Autodesk Inventor part; units mm, degrees
ref_plane "YZ Plane" through (0, 0, 0) normal (1, 0, 0) x (0, 1, 0)
ref_plane "XZ Plane" through (0, 0, 0) normal (0, 1, 0) x (-1, 0, 0)
ref_plane "XY Plane" through (0, 0, 0) normal (0, 0, 1) x (1, 0, 0)
sketch "Sketch1" plane through (0, 0, 0) normal (0, 1, 0) x (-1, 0, 0)
  circle A0 centre (0, 0) radius 66.5
  circle A1 centre (0, 0) radius 15
  dimension "d0" = 133
  dimension "d3" = 30
extrude "Extrusion2" add sketch "Sketch1" along normal blind 3
sketch "Sketch3" plane through (0, 3, 0) normal (0, 1, 0) x (1, 0, 0)
  circle A0 centre (0, 0) radius 66.5
  circle A1 centre (0, 0) radius 68.5
  dimension "d6" = 133
  dimension "d7" = 137
extrude "Extrusion3" add sketch "Sketch3" against normal blind 17
sketch "Sketch4" plane through (0, 0, 0) normal (0, -1, 0) x (1, 0, 0)
  circle A0 centre (0, 0) radius 15
  circle A1 centre (0, 0) radius 39
  line L0 (10.6103, -10.6029) -> (27.5808, -27.5735)
  line L1 (39, 0) -> (15, 0)
  circle A2 centre (0, 0) radius 15
  line L2 (27.7885, -27.3642) -> (10.8166, -10.3923)
  dimension "d10" = 30
  dimension "d11" = 24
extrude "Extrusion4" cut sketch "Sketch4" against normal blind 1.5 contours L1 A1 L2 A0 | A0 L2 A1 L0
mirror "Mirror1" about plane through (0, 0, 0) normal (0, 0, 1) of "Extrusion4"
fillet "Fillet1" radius 6 1 edges at (-68.5, 3, 0)
fillet "Fillet2" radius 2 1 edges at (-66.5, 0, 0)
properties part number "DireccionBase"
Geometry: final body of the model. Coordinates: model frame, mm. A direction names the side the tool comes from. Give positions to 0.01 mm unless a question says otherwise; leave off trailing zeros. Loops run counter-clockwise (first coordinate to the right, second up) from the corner with the lowest first, then second, coordinate; pieces in that order, holes last. Notation, with made-up numbers: (38, -13.75) -> (55, -13.75) arc R28 cw to (55, 4.25) -> close; hole circle Ø9 at (68.5, 78.25). An arc over 180 degrees is marked (long way). Put each result on its own line as item: value.
1. Set-up query: faces 4 (the cylindrical face through (-13.856, 1.479, 5.745)), 5 (the flat face through (25, 1.5, 0)). Return all of +Z, -Z, +X, -X, +Y, -Y with unobstructed straight access to the full face (end or side cutting, diameter ignored); none if empty.
Taken from the geometry:
face 4: +Y, -Y
face 5: -Y
2. Pin query (flat end, axial travel): P1, Ø8, axis at x = -37, y = -2.5, coming from the +Z side; P2, Ø5, axis at x = -39.5, y = -4.5, coming from the +Z side; P3, Ø3, axis at x = 40.5, y = -2, coming from the +Z side; P4, Ø18, axis at x = 0, z = 0, coming from the -Y side. Return the tip coordinate at first contact, or that it passes through.
Taken from the geometry:
P1: stops at z = 60.02
P2: stops at z = 57.65
P3: stops at z = 56.24
P4: passes through
3. Ray query, line 1 along X through (y, z) = (-5, 0); line 2 along Y through (x, z) = (37, -10.5). Return the intervals inside material, ascending. Write a range as [from, to].
Taken from the geometry:
line 1: x = [-68.5, -66.5], [66.5, 68.5]
line 2: y = [1.5, 3]
4. Cut plane B-B (x = 0). Return the cut outline in (y, z), plus the area to 3 significant figures.
Taken from the geometry:
outline: (-14, -68.5) -> (-3, -68.5) arc R6 ccw to (3, -62.5) -> (3, -15) -> (0, -15) -> (0, -64.5) arc R2 cw to (-2, -66.5) -> (-14, -66.5) -> close; (-14, 66.5) -> (-2, 66.5) arc R2 cw to (0, 64.5) -> (0, 15) -> (3, 15) -> (3, 62.5) arc R6 ccw to (-3, 68.5) -> (-14, 68.5) -> close
area: 363 mm2
5. Cut plane A-A (z = 0). Return the cut outline in (x, y), plus the area to 3 significant figures.
Taken from the geometry:
outline: (-68.5, -14) -> (-66.5, -14) -> (-66.5, -2) arc R2 cw to (-64.5, 0) -> (-15, 0) -> (-15, 3) -> (-62.5, 3) arc R6 ccw to (-68.5, -3) -> close; (15, 1.5) -> (39, 1.5) -> (39, 0) -> (64.5, 0) arc R2 cw to (66.5, -2) -> (66.5, -14) -> (68.5, -14) -> (68.5, -3) arc R6 ccw to (62.5, 3) -> (15, 3) -> close
area: 327 mm2
6. Cut plane C-C (y = -4.75). Return the cut outline in (x, z), plus the area to 3 significant figures.
Taken from the geometry:
outline: circle Ø137 at (0, 0); hole circle Ø133 at (0, 0)
area: 848 mm2
7. Pull-direction query (X, two-part tool) for faces 1 (the flat face through (0.9, 0, 15.2)), 2 (the flat face through (-13, 3, -13)), 3 (the cylindrical face through (65.337, -8.423, -20.576)); classes: released by +X, released by -X, zero draft, split by the parting line, or undercut.
Taken from the geometry:
face 1: undercut
face 2: zero draft
face 3: split by the parting line
